Source: CAD feature listing. Evaluate the final solid. Frame: model axes, mm. Face numbers are marked on the shaded views. Give positions to 0.01 mm unless a question says otherwise; leave off trailing zeros. Write each loop counter-clockwise with the first axis right and the second up, starting at its lowest first coordinate (ties: lowest second). Pieces come first, ordered by that corner, then holes. Notation, with made-up numbers: M -11,20 L 12,20 A27 cw 12,54 Z; hole C -17,59 d11. An arc over 180 degrees is marked long. Return JSON: item names as keys, results as strings.
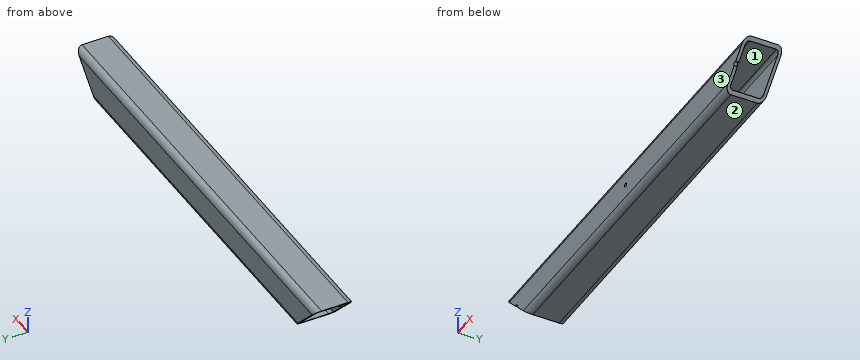
```python
from build123d import *

# Parameters (mm, degrees)
TUBE_SQUARE_40_X_40_X_3_2_9_DEPTH = 460
CUT_EXTRUDE1_DEPTH                = 463.168800332
SKETCH15_R                        = 2
CUT_EXTRUDE4_DEPTH                = 461.868744872


with BuildPart() as part:
    # Sketch12 → Tube (square) 40 X 40 X 3.2(9) (new body)
    with BuildSketch(Plane(origin=(0, 0, 0), x_dir=(0, 0, -1), z_dir=(1, 0, 0))):
        with BuildLine():
            Line((-13.6, -20), (13.6, -20))
            ThreePointArc((13.6, -20), (18.1254834, -18.1254834), (20, -13.6))
            Line((20, -13.6), (20, 13.6))
            ThreePointArc((20, 13.6), (18.1254834, 18.1254834), (13.6, 20))
            Line((13.6, 20), (-13.6, 20))
            ThreePointArc((-13.6, 20), (-18.1254834, 18.1254834), (-20, 13.6))
            Line((-20, 13.6), (-20, -13.6))
            ThreePointArc((-20, -13.6), (-18.1254834, -18.1254834), (-13.6, -20))
        make_face()
        with BuildLine():
            Line((-13.6, -16.8), (13.6, -16.8))
            ThreePointArc((13.6, -16.8), (15.8627417, -15.8627417), (16.8, -13.6))
            Line((16.8, -13.6), (16.8, 13.6))
            ThreePointArc((16.8, 13.6), (15.8627417, 15.8627417), (13.6, 16.8))
            Line((13.6, 16.8), (-13.6, 16.8))
            ThreePointArc((-13.6, 16.8), (-15.8627417, 15.8627417), (-16.8, 13.6))
            Line((-16.8, 13.6), (-16.8, -13.6))
            ThreePointArc((-16.8, -13.6), (-15.8627417, -15.8627417), (-13.6, -16.8))
        make_face(mode=Mode.SUBTRACT)
    extrude(amount=TUBE_SQUARE_40_X_40_X_3_2_9_DEPTH)

    # Sketch13 → Cut-Extrude1 (cut, through all)
    with BuildSketch(Plane(origin=(0, 20, 0), x_dir=(1, 0, 0), z_dir=(0, 1, 0))):
        Polygon((460, 20), (460, -20), (420, 20), align=None)
        Polygon((0, 20), (0, -20), (40, 20), align=None)
    extrude(amount=-CUT_EXTRUDE1_DEPTH, mode=Mode.SUBTRACT)

    # Sketch15 → Cut-Extrude4 (cut, through all)
    with BuildSketch(Plane(origin=(0, 0, 0), x_dir=(1, 0, 0), z_dir=(0, 1, 0))):
        with Locations((440, 0)):
            Circle(SKETCH15_R)
        with Locations(Location((230, 0, 0), (0, 0, 270))):
            Circle(SKETCH15_R)
        with Locations((20, 0)):
            Circle(SKETCH15_R)
    extrude(amount=-CUT_EXTRUDE4_DEPTH, mode=Mode.SUBTRACT)


solid = part.part
```
1) Cut plane A-A, the plane z = -6. Return the cut outline in (x, y), then the cut area to 3 significant figures.
Numbers:
{"outline": "M 26,-20 L 434,-20 L 434,-16.8 L 26,-16.8 Z; M 26,16.8 L 434,16.8 L 434,20 L 26,20 Z", "area": "2,610 mm²"}
2) Cut plane C-C, the plane y = 3.5. Return the cut outline in (x, z), then the cut area to 3 significant figures.
Numbers:
{"outline": "M 0,20 L 3.2,16.8 L 456.8,16.8 L 460,20 Z; M 36.8,-16.8 L 40,-20 L 420,-20 L 423.2,-16.8 Z", "area": "2,690 mm²"}
3) Line query: line 1 (Z direction, x = 283.5, y = -6); line 2 (X direction, y = -17, z = 0). Output: solid intervals per line, ascending. Write a range as [from, to].
Numbers:
{"line 1": "z = [-20, -16.8], [16.8, 20]", "line 2": "x = [22, 228], [232, 438]"}
4) Draft query along Y for the marked faces 1, 2 and 3. Return one class per face: released by +Y, released by -Y, zero draft, split by the parting line, or undercut.
Numbers:
{"face 1": "undercut", "face 2": "zero draft", "face 3": "released by -Y"}
5) Cut plane B-B, the plane x = 324. Return the cut outline in (y, z).
Numbers:
{"outline": "M -20,-13.6 A6.4 ccw -13.6,-20 L 13.6,-20 A6.4 ccw 20,-13.6 L 20,13.6 A6.4 ccw 13.6,20 L -13.6,20 A6.4 ccw -20,13.6 Z; hole M -16.8,-13.6 A3.2 ccw -13.6,-16.8 L 13.6,-16.8 A3.2 ccw 16.8,-13.6 L 16.8,13.6 A3.2 ccw 13.6,16.8 L -13.6,16.8 A3.2 ccw -16.8,13.6 Z"}
